For this review, take the finished solid that the model builds, in its own axes (mm). A direction names the side the tool comes from. Round coordinates to 2 decimals unless told otherwise and drop trailing zeros. Loops run counter-clockwise (first coordinate to the right, second up) from the corner with the lowest first, then second, coordinate; pieces in that order, holes last.
1. Consider section C-C on x = 0. State the section outline as (y, z) points, then the cut area to 3 significant figures.
2. Clearance check with flat-ended pins moving along their axes: pin 1 Ø8 at (x, z) = (-22, 13) entering from -Y; pin 2 Ø4 at (y, z) = (4.5, 19.5) entering from +X; pin 3 Ø6 at (y, z) = (-6.5, 17) entering from +X; pin 4 Ø5 at (x, y) = (-50, 0) entering from +Z. State where each tip first meets the part, or that it passes through.
3. Consider section D-D on z = 18.25. State the section outline as (x, y) points, then the cut area to 3 significant figures.
4. To check wall thickness, follow line 1 along Y through (x, z) = (30, 4); line 2 along Z through (x, y) = (65, -13.5); line 3 along X through (y, z) = (5, 18.5). State the ranges of each line that lie inside material, in increasing order.
5. Consider section A-A on x = -50. State the section outline as (y, z) points, then the cut area to 3 significant figures.
6. Consider section B-B on y = 8. State the section outline as (x, z) points, then the cut area to 3 significant figures.
7. Tool access review of faces 1 (the cylindrical face through (11.923, 3.755, 17.395)), 2 (the flat face through (0, 0, 25)): name each direction out of +Z, -Z, +X, -X, +Y, -Y from which nothing blocks a thin tool from reaching the whole face with its end or side.
from build123d import *

# Parameters (mm, degrees)
F0_W     = 150
F0_H     = 50
F1_DEPTH = 10
F2_R     = 12.5
F3_DEPTH = 15
F5_D     = 4.2


with BuildPart() as f1:
    # F0 (on Top) → F1 (new body)
    with BuildSketch(Plane.XY):
        Rectangle(F0_W, F0_H)
    extrude(amount=F1_DEPTH)

    # F2 (on face) → F3 (join)
    with BuildSketch(Plane.XY.offset(10)):
        Circle(F2_R)
    extrude(amount=F3_DEPTH)

    # F5 (through all)
    with Locations(Plane.XY.offset(10)):
        with Locations((-50, 0), (30, 0)):
            Hole(F5_D / 2)


solid = f1.part
Resolved:
1. outline: (-25, 0) - (25, 0) - (25, 10) - (12.5, 10) - (12.5, 25) - (-12.5, 25) - (-12.5, 10) - (-25, 10) - close
1. area: 875 mm2
2. pin 1: stops at y = -25
2. pin 2: stops at x = 12.25
2. pin 3: stops at x = 12
2. pin 4: stops at z = 10
3. outline: circle Ø25 at (0, 0)
3. area: 491 mm2
4. line 1: y = -25 to -2.1, 2.1 to 25
4. line 2: z = 0 to 10
4. line 3: x = -11.46 to 11.46
5. outline: (-25, 0) - (-2.1, 0) - (-2.1, 10) - (-25, 10) - close; (2.1, 0) - (25, 0) - (25, 10) - (2.1, 10) - close
5. area: 458 mm2
6. outline: (-75, 0) - (75, 0) - (75, 10) - (9.6, 10) - (9.6, 25) - (-9.6, 25) - (-9.6, 10) - (-75, 10) - close
6. area: 1,790 mm2
7. face 1: +Z
7. face 2: +Z, +X, -X, +Y, -Y
